from build123d import *

# Parameters (mm, degrees)
RESSALTO_EXTRUS_O2_DEPTH = 20
ESBO_O3_R                = 14
BOSS_EXTRUDE1_DEPTH      = 10
SKETCH2_R                = 1
BOSS_EXTRUDE2_DEPTH      = 5
CUT_EXTRUDE2_DEPTH       = 20


with BuildPart() as part:
    # Esboço1 → Ressalto-extrusão2 (new body)
    with BuildSketch(Plane(origin=(0, 0, 0), x_dir=(1, 0, 0), z_dir=(0, 1, 0))):
        with BuildLine():
            ThreePointArc((-12.5, -21.650635095), (0, -25), (12.5, -21.650635095))
            ThreePointArc((12.5, -21.650635095), (21.650635095, -12.5), (25, 0))
            ThreePointArc((25, 0), (-12.5, 21.650635095), (-12.5, -21.650635095))
        make_face()
    extrude(amount=RESSALTO_EXTRUS_O2_DEPTH)

    # Esboço3 → Boss-Extrude1 (add)
    with BuildSketch(Plane(origin=(0, 20, 0), x_dir=(1, 0, 0), z_dir=(0, 1, 0))):
        with Locations(Location((0, 0, 0), (0, 0, 270))):
            Circle(ESBO_O3_R)
    extrude(amount=BOSS_EXTRUDE1_DEPTH)

    # Sketch2 → Boss-Extrude2 (add)
    with BuildSketch(Plane(origin=(0, 30, 0), x_dir=(1, 0, 0), z_dir=(0, 1, 0))):
        with Locations(Location((0, 0, 0), (0, 0, 270))):
            Circle(SKETCH2_R)
        with Locations(Location((10.5, 0, 0), (0, 0, 270))):
            Circle(SKETCH2_R)
    extrude(amount=BOSS_EXTRUDE2_DEPTH)

    # Sketch3 → Cut-Extrude2 (cut)
    with BuildSketch(Plane(origin=(0, 20, 0), x_dir=(1, 0, 0), z_dir=(0, 1, 0))):
        with BuildLine():
            Line((8.185723081, -18.248121483), (6.13929231, -13.686091112))
            ThreePointArc((6.13929231, -13.686091112), (15, 0), (6.13929231, 13.686091112))
            Line((6.13929231, 13.686091112), (8.185723081, 18.248121483))
            ThreePointArc((8.185723081, 18.248121483), (20, 0), (8.185723081, -18.248121483))
        make_face()
    extrude(amount=-CUT_EXTRUDE2_DEPTH, mode=Mode.SUBTRACT)


solid = part.part
Check sheet for the modelled part. Datum: model origin and axes. Units: mm. A direction names the side the tool comes from. Round coordinates to 2 decimals unless told otherwise and drop trailing zeros. Loops run counter-clockwise (first coordinate to the right, second up) from the corner with the lowest first, then second, coordinate; pieces in that order, holes last.
1. Mould release check, pull along X, two halves, no side actions. Record for faces 4 (the cylindrical face through (-13.67, 24.93, -3.03)), 5 (the flat face through (11, 35, 0)), 6 (the cylindrical face through (15, 10, 0)): released by +X, released by -X, zero draft, split by the parting line, or undercut.
2. Gauge pin test, flat ends, axial feed: pin 1 Ø3 at (x, z) = (8.5, 14) entering from +Y; pin 2 Ø12 at (y, z) = (27.5, -9) entering from -X; pin 3 Ø2 at (y, z) = (10.5, -13) entering from -X. Record the tip position at first contact, or that the pin passes through.
3. Set-up check for faces 1 (the flat face through (7.15, 10.14, -15.94)), 2 (the flat face through (0, 0, 0)), 3 (the cylindrical face through (-1, 32, 0)): record each of +Z, -Z, +X, -X, +Y, -Y from which the full face is reachable in a straight line by a thin tool's end or side.
4. Sectioned sample at C-C on z = 2.5. Record the boundary of the cut face in (x, y), and give its area (3 significant figures).
5. Sectioned sample at D-D on x = 0. Record the boundary of the cut face in (y, z).
6. Sectioned sample at A-A on y = 10. Record the boundary of the cut face in (x, z).
7. Sectioned sample at B-B on x = 16. Record the boundary of the cut face in (y, z), and give its area (3 significant figures).
8. Scan lines: probe 1 along Y at (x, z) = (-14, 8.5); probe 2 along Z at (x, y) = (-0.5, 25.5); probe 3 along Y at (x, z) = (13.5, -2.5). Record each from-to range of solid material in increasing order.
Recorded:
1. face 4: split by the parting line
1. face 5: zero draft
1. face 6: undercut
2. pin 1: stops at y = 20
2. pin 2: stops at x = -13.67
2. pin 3: stops at x = -21.93
3. face 1: +Y, -Y
3. face 2: +Z, -Z, +X, -X, -Y
3. face 3: +Y
4. outline: (-24.87, 0) - (14.79, 0) - (14.79, 20) - (13.77, 20) - (13.77, 30) - (-13.77, 30) - (-13.77, 20) - (-24.87, 20) - close; (19.84, 0) - (24.87, 0) - (24.87, 20) - (19.84, 20) - close
4. area: 1,170 mm2
5. outline: (0, -25) - (20, -25) - (20, -14) - (30, -14) - (30, -1) - (35, -1) - (35, 1) - (30, 1) - (30, 14) - (20, 14) - (20, 25) - (0, 25) - close
6. outline: circle Ø50 at (0, 0); hole (6.14, -13.69) - (8.19, -18.25) arc R20 ccw to (8.19, 18.25) - (6.14, 13.69) arc R15 cw to start
7. outline: (0, -19.21) - (20, -19.21) - (20, -12) - (0, -12) - close; (0, 12) - (20, 12) - (20, 19.21) - (0, 19.21) - close
7. area: 288 mm2
8. probe 1: y = 0 to 20
8. probe 2: z = -13.99 to 13.99
8. probe 3: y = 0 to 30
